from build123d import *

# Parameters (mm, degrees)
CROQUIS2_R              = 1.5
SALIENTE_EXTRUIR1_DEPTH = 4
CROQUIS3_R              = 5
CROQUIS3_R_2            = 2.5
SALIENTE_EXTRUIR2_DEPTH = 13


with BuildPart() as part:
    # Croquis2 → Saliente-Extruir1 (new body)
    with BuildSketch(Plane.XY):
        Polygon((2.886751346, 5), (-2.886751346, 5), (-5.773502692, 0), (-2.886751346, -5), (2.886751346, -5), (5.773502692, 0), align=None)
        Circle(CROQUIS2_R, mode=Mode.SUBTRACT)
    extrude(amount=SALIENTE_EXTRUIR1_DEPTH)

    # Croquis3 → Saliente-Extruir2 (add)
    with BuildSketch(Plane(origin=(0, 0, 0), x_dir=(-1, 0, 0), z_dir=(0, 0, -1))):
        Circle(CROQUIS3_R)
        Circle(CROQUIS3_R_2, mode=Mode.SUBTRACT)
    extrude(amount=SALIENTE_EXTRUIR2_DEPTH)


solid = part.part
Verification items for the finished model (mm, model axes). A direction names the side the tool comes from. Give positions to 0.01 mm unless a question says otherwise; leave off trailing zeros. Loops run counter-clockwise (first coordinate to the right, second up) from the corner with the lowest first, then second, coordinate; pieces in that order, holes last.
1) Sectioned sample at C-C, the plane x = 1.75. Enter the section's corners in (y, z), then the cut area to 3 significant figures.
2) Draft check along Y on faces 1 (the flat face through (4.35, 2.465, 1.972)), 2 (the cylindrical face through (-1.5, 0.07, 1.97)), 3 (the flat face through (5.2, 0, 0)), 4 (the flat face through (2, 0, 0)). Enter one of: pulls with the +Y half, pulls with the -Y half, needs draft (parallel to the pull), parting line crosses it, or undercut.
3) Sectioned sample at B-B, the plane y = 1. Enter the section's corners in (x, z).
4) Depth check by flat-ended pin: pin 1 Ø2 at (y, z) = (-2, -8) entering from +X; pin 2 Ø2 at (y, z) = (-3.5, -10.5) entering from -X; pin 3 Ø3 at (x, z) = (2, -2.5) entering from +Y. Enter the tip coordinate at first touch or a pass-through.
5) Set-up check for faces 5 (the cylindrical face through (0.54, -2.44, -6.41)), 6 (the flat face through (-2.7, -4.5, 0)), 7 (the flat face through (-2.7, 4.5, 0)), 8 (the flat face through (2.6, 4.5, 0)): record each of +Z, -Z, +X, -X, +Y, -Y from which the full face is reachable in a straight line by a thin tool's end or side.
6) Thickness scan on line 1 along Y through (x, z) = (0, -8); line 2 along Y through (x, z) = (0, 0.9); line 3 along Z through (x, y) = (-0.5, 2.25). Record the ranges inside material, lowest first.
7) Sectioned sample at A-A, the plane z = 1.25. Enter the section's corners in (x, y).
Answers:
1. outline: (-5, 0) - (-4.68, 0) - (-4.68, -13) - (-1.79, -13) - (-1.79, 0) - (1.79, 0) - (1.79, -13) - (4.68, -13) - (4.68, 0) - (5, 0) - (5, 4) - (-5, 4) - close
1. area: 115 mm2
2. face 1: pulls with the +Y half
2. face 2: undercut
2. face 3: needs draft
2. face 4: undercut
3. outline: (-5.2, 0) - (-4.9, 0) - (-4.9, -13) - (-2.29, -13) - (-2.29, 0) - (-1.12, 0) - (-1.12, 4) - (-5.2, 4) - close; (1.12, 0) - (2.29, 0) - (2.29, -13) - (4.9, -13) - (4.9, 0) - (5.2, 0) - (5.2, 4) - (1.12, 4) - close
4. pin 1: stops at x = 4.9
4. pin 2: stops at x = -4.33
4. pin 3: stops at y = 4.97
5. face 5: -Z
5. face 6: -Z, -X, -Y
5. face 7: -Z, -X, +Y
5. face 8: -Z, +X, +Y
6. line 1: y = -5 to -2.5, 2.5 to 5
6. line 2: y = -5 to -1.5, 1.5 to 5
6. line 3: z = 0 to 4
7. outline: (-5.77, 0) - (-2.89, -5) - (2.89, -5) - (5.77, 0) - (2.89, 5) - (-2.89, 5) - close; hole circle Ø3 at (0, 0)
